The listing builds one solid part. Answer for the finished solid, in the listing's coordinates (mm). A direction names the side the tool comes from. Round coordinates to 2 decimals unless told otherwise and drop trailing zeros. Write each loop counter-clockwise with the first axis right and the second up, starting at its lowest first coordinate (ties: lowest second). Pieces come first, ordered by that corner, then holes. Notation, with made-up numbers: M 44,7 L 99,7 A20 cw 99,46 Z; hole C 60.5,8 d2. An arc over 180 degrees is marked long. Put each result on its own line as item: value. Start each with the question number.
```python
from build123d import *

# Parameters (mm, degrees)
BOSS_EXTRUDE1_DEPTH = 2.032
BOSS_EXTRUDE2_DEPTH = 2.54
FILLET2_R           = 1.27


with BuildPart() as part:
    # Sketch1 → Boss-Extrude1 (new body)
    with BuildSketch(Plane(origin=(0, 0, 0), x_dir=(1, 0, 0), z_dir=(0, 1, 0))):
        Polygon((27.94, 0), (13.97, 24.196749782), (-13.97, 24.196749782), (-27.94, 0), (-13.97, -24.196749782), (13.97, -24.196749782), align=None)
    extrude(amount=BOSS_EXTRUDE1_DEPTH)

    # Sketch2 → Boss-Extrude2 (add)
    with BuildSketch(Plane(origin=(0, 2.032, 0), x_dir=(1, 0, 0), z_dir=(0, 1, 0))):
        Polygon((11.564989719, -20.031149782), (3.944989719, -20.031149782), (5.118165466, -22.063149782), (12.738165466, -22.063149782), (16.548165466, -15.464036205), (15.374989719, -13.432036205), align=None)
        Polygon((-23.129979437, 0), (-19.319979437, 6.599113577), (-21.666330931, 6.599113577), (-25.476330931, 0), (-21.666330931, -6.599113577), (-19.319979437, -6.599113577), align=None)
        Polygon((5.118165466, 22.063149782), (3.944989719, 20.031149782), (11.564989719, 20.031149782), (15.374989719, 13.432036205), (16.548165466, 15.464036205), (12.738165466, 22.063149782), align=None)
    extrude(amount=BOSS_EXTRUDE2_DEPTH)

    # Fillet2
    fillet2_edges = [part.edges().sort_by_distance(p)[0] for p in [
        (15.374989719, 3.302, -13.432036205),
        (3.944989719, 3.302, -20.031149782),
        (15.374989719, 3.302, 13.432036205),
        (3.944989719, 3.302, 20.031149782),
        (-19.319979437, 3.302, 6.599113577),
        (-19.319979437, 3.302, -6.599113577),
    ]]
    fillet(fillet2_edges, radius=FILLET2_R)


solid = part.part
```
Item 1: Section A-A (y = 3.6) is taken. Give the vertices of the cut face in (x, z), and give its area (3 significant figures).
Item 2: Which of the six approach directions +Z, -Z, +X, -X, +Y, -Y give full straight-line access (tool end or side, diameter ignored) to faces 5 (the flat face through (12.9, 3.28, -17.72)), 6 (the flat face through (0, 2.032, 0)), 7 (the flat face through (9, 3, 22.063)), 8 (the flat face through (-23.6, 3.28, 3.25)), 9 (the cylindrical face through (-20.43, 3.32, 5.98))?
Item 3: Determine the mould class of faces 1 (the flat face through (14.67, 3.28, -18.72)), 2 (the flat face through (14.616, 3.284, 18.81)), 3 (the cylindrical face through (5.036, 3.32, -20.682)), 4 (the flat face through (12.94, 3.28, 17.65)) for opening direction Z: released by +Z, released by -Z, zero draft, split by the parting line, or undercut.
Item 4: Section D-D (y = 0.65) is taken. Give the vertices of the cut face in (x, z), and give its area (3 significant figures).
Item 5: Consider line 1 along Y through (x, z) = (9.5, 8); line 2 along Z through (x, y) = (-22, 2.9); line 3 along Z through (x, y) = (11.5, 3.35). Determine where each line is inside the solid, lowest interval first. Write a range as [from, to].
Item 6: Section B-B (x = 9) is taken. Give the vertices of the cut face in (y, z).
Item 7: Flat-ended cylindrical pins translate along their axes: pin 1 (2 mm diameter, centred on x = 10.5, y = 3.5, fed in from +Z); pin 2 (3 mm diameter, centred on x = -12.5, z = -6, fed in from +Y); pin 3 (0.8 mm diameter, centred on x = 9.5, y = 3.5, fed in from -Z). Find the tip coordinate at first contact, or state that the pin passes through.
Item 8: Section C-C (z = 1.5) is taken. Give the vertices of the cut face in (x, y), and give its area (3 significant figures).
Output values:
1. outline: M -25.48,0 L -21.67,-6.6 L -21.52,-6.6 A1.27 ccw -20.42,-4.69 L -23.13,0 L -20.42,4.69 A1.27 ccw -21.52,6.6 L -21.67,6.6 Z; M 5.04,-21.94 L 5.12,-22.06 L 12.74,-22.06 L 16.55,-15.46 L 16.47,-15.34 A1.27 ccw 14.28,-15.34 L 11.56,-20.03 L 6.14,-20.03 A1.27 ccw Z; M 5.04,21.94 A1.27 ccw 6.14,20.03 L 11.56,20.03 L 14.28,15.34 A1.27 ccw 16.47,15.34 L 16.55,15.46 L 12.74,22.06 L 5.12,22.06 Z
1. area: 86.3 mm^2
2. face 5: -X, +Y
2. face 6: +Y
2. face 7: +Z, +X, -X, +Y
2. face 8: +Z, -X, +Y
2. face 9: +X, +Y
3. face 1: released by -Z
3. face 2: released by +Z
3. face 3: undercut
3. face 4: undercut
4. outline: M -27.94,0 L -13.97,-24.2 L 13.97,-24.2 L 27.94,0 L 13.97,24.2 L -13.97,24.2 Z
4. area: 2,030 mm^2
5. line 1: y = [0, 2.03]
5. line 2: z = [-6.02, -1.96], [1.96, 6.02]
5. line 3: z = [-22.06, -20.03], [20.03, 22.06]
6. outline: M 0,-24.2 L 2.03,-24.2 L 2.03,-22.06 L 4.57,-22.06 L 4.57,-20.03 L 2.03,-20.03 L 2.03,20.03 L 4.57,20.03 L 4.57,22.06 L 2.03,22.06 L 2.03,24.2 L 0,24.2 Z
7. pin 1: stops at z = 22.06
7. pin 2: stops at y = 2.03
7. pin 3: stops at z = -22.06
8. outline: M -27.07,0 L 27.07,0 L 27.07,2.03 L -22.26,2.03 L -22.26,4.57 L -24.61,4.57 L -24.61,2.03 L -27.07,2.03 Z
8. area: 116 mm^2
